Part model, mm, in its own coordinate system. Face numbers are marked on the shaded views. A direction names the side the tool comes from. Give positions to 0.01 mm unless a question says otherwise; leave off trailing zeros. Order: outer loops, then holes, each group sorted by start corner. A loop starts at its lowest first (then second) coordinate and runs counter-clockwise, first axis right, second up.
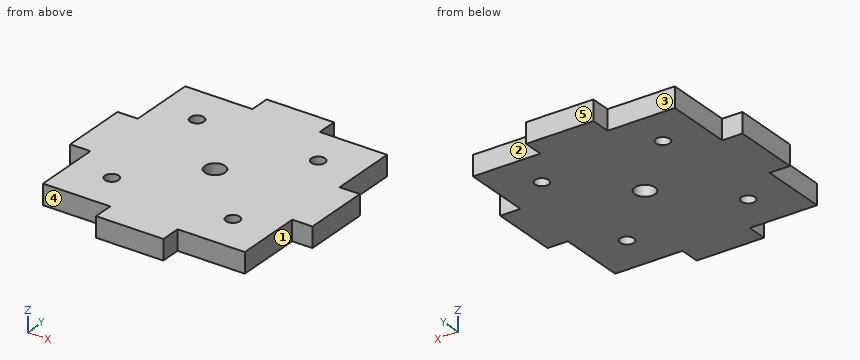
from build123d import *

# Parameters (mm, degrees)
BOSS_EXTRUDE1_DEPTH = 5
CAVITY1_OUTLINE_R   = 2.5
CAVITY1_OUTLINE_R_2 = 1.7
CAVITY1_DEPTH       = 5


# Read off the part's stored shape, not the designer's step: Cavity1
with BuildPart() as part:
    # Sketch1 → Boss-Extrude1 (new body)
    with BuildSketch(Plane.XY):
        Polygon((-22.75, 8.333333333), (-22.75, 25), (-6.083333333, 25), (-6.083333333, 30), (10.583333333, 30), (10.583333333, 25), (27.25, 25), (27.25, 8.333333333), (32.25, 8.333333333), (32.25, -8.333333333), (27.25, -8.333333333), (27.25, -25), (10.583333333, -25), (10.583333333, -30), (-6.083333333, -30), (-6.083333333, -25), (-22.75, -25), (-22.75, -8.333333333), (-27.75, -8.333333333), (-27.75, 8.333333333), align=None)
    extrude(amount=BOSS_EXTRUDE1_DEPTH)

    # Cavity1 outline → Cavity1 (cut)
    with BuildSketch(Plane.XY):
        with Locations((2.25, 0)):
            Circle(CAVITY1_OUTLINE_R)
        with Locations((-12.75, 15)):
            Circle(CAVITY1_OUTLINE_R_2)
        with Locations((17.25, 15)):
            Circle(CAVITY1_OUTLINE_R_2)
        with Locations((17.25, -15)):
            Circle(CAVITY1_OUTLINE_R_2)
        with Locations((-12.75, -15)):
            Circle(CAVITY1_OUTLINE_R_2)
    extrude(amount=CAVITY1_DEPTH, mode=Mode.SUBTRACT)


solid = part.part
Item 1: Which spindle directions (+Z, -Z, +X, -X, +Y, -Y) get a long thin tool onto all of the face, cutting with end or side? Do the marked faces 1, 2, 3, 4 and 5. Say none if no direction does.
Item 2: Band-saw the part on A-A on y = 0. List the corners of the cut face in (x, z).
Item 3: Band-saw the part on D-D on x = 17.25. List the corners of the cut face in (y, z), plus the area to 3 significant figures.
Item 4: Band-saw the part on C-C on y = 15. List the corners of the cut face in (x, z), plus the area to 3 significant figures.
Item 5: Drop flat-ended pins along their axis: P1, Ø4, axis at x = 2.25, y = 0, coming from the +Z side; P2, Ø4, axis at x = -12.75, y = -15, coming from the -Z side; P3, Ø1.5, axis at x = 18.5, z = 1.5, coming from the -Y side; P4, Ø1.5, axis at y = 17, z = 3, coming from the +X side. Give the stop position or say it passes through.
Item 6: Band-saw the part on B-B on x = 2.25. List the corners of the cut face in (y, z).
Item 7: Drill centre lines: probe 1 along Y at (x, z) = (-12.75, 3.15); probe 2 along Y at (x, z) = (-21, 2.4); probe 3 along Y at (x, z) = (28, 2.9). Where is each one in solid material? Low to high.
Working result:
1. face 1: +Z, -Z, +X, -Y
1. face 2: +Z, -Z, +X, +Y
1. face 3: +Z, -Z, -X, +Y
1. face 4: +Z, -Z, -X, -Y
1. face 5: +Z, -Z, +X, -X, +Y
2. outline: (-27.75, 0) - (-0.25, 0) - (-0.25, 5) - (-27.75, 5) - close; (4.75, 0) - (32.25, 0) - (32.25, 5) - (4.75, 5) - close
3. outline: (-25, 0) - (-16.7, 0) - (-16.7, 5) - (-25, 5) - close; (-13.3, 0) - (13.3, 0) - (13.3, 5) - (-13.3, 5) - close; (16.7, 0) - (25, 0) - (25, 5) - (16.7, 5) - close
3. area: 216 mm2
4. outline: (-22.75, 0) - (-14.45, 0) - (-14.45, 5) - (-22.75, 5) - close; (-11.05, 0) - (15.55, 0) - (15.55, 5) - (-11.05, 5) - close; (18.95, 0) - (27.25, 0) - (27.25, 5) - (18.95, 5) - close
4. area: 216 mm2
5. P1: passes through
5. P2: stops at z = 0
5. P3: stops at y = -25
5. P4: stops at x = 27.25
6. outline: (-30, 0) - (-2.5, 0) - (-2.5, 5) - (-30, 5) - close; (2.5, 0) - (30, 0) - (30, 5) - (2.5, 5) - close
7. probe 1: y = -25 to -16.7, -13.3 to 13.3, 16.7 to 25
7. probe 2: y = -25 to 25
7. probe 3: y = -8.33 to 8.33
